Source: three-view drawing plus pictorial views. Frame: mm from the lowest corner of the part. A direction names the side the tool comes from. Give positions to 0.01 mm unless a question says otherwise; leave off trailing zeros. Write each loop counter-clockwise with the first axis right and the second up, starting at its lowest first coordinate (ties: lowest second). Pieces come first, ordered by that corner, then holes. Notation, with made-up numbers: (-12.5, -9.75) - (30.5, -9.75) arc R20 ccw to (30.5, 26.25) - close; hole circle Ø1 at (56, 11.5). An arc over 180 degrees is marked (long way). One line per question, with ' | ' between items. Start each with the question number.
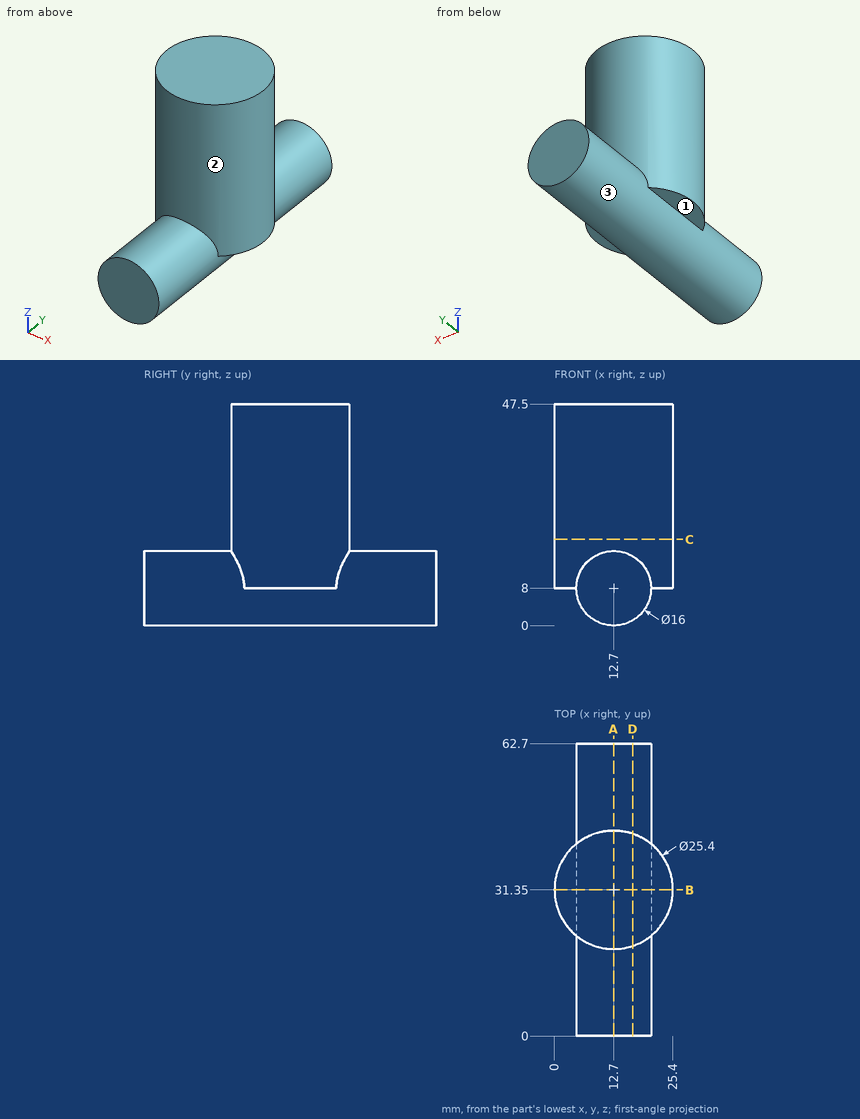
1) First-contact query: pin 1 Ø1.4 at (x, y) = (24, 28.5) entering from -Z; pin 2 Ø1.5 at (x, z) = (3.5, 24) entering from +Y; pin 3 Ø1.5 at (x, z) = (19, 16.5) entering from +Y. Flat tips, straight axial feed; report the tip coordinate or a pass-through.
2) Section B-B, the plane y = 31.35. Output: boundary loops of the cut face in (x, z), plus the area to 3 significant figures.
3) Reachability of the marked faces 1, 2 and 3 from +Z, -Z, +X, -X, +Y, -Y: full face, straight path, thin tool, end or side. Return the list, or none.
4) Section A-A, the plane x = 12.7. Output: boundary loops of the cut face in (y, z).
5) Section C-C, the plane z = 18.5. Output: boundary loops of the cut face in (x, y).
6) Section D-D, the plane x = 16.75. Output: boundary loops of the cut face in (y, z).
7) Line query: L1, parallel to X at y = 31.5, z = 11; L2, parallel to Y at x = 20.25, z = 41; L3, parallel to Z at x = 9, y = 45.5. Output: solid intervals per line, ascending.
Answer key:
1) pin 1: z = 8 | pin 2: y = 40.83 | pin 3: y = 42.77
2) outline: (0, 8) - (4.7, 8) arc R8 ccw to (20.7, 8) - (25.4, 8) - (25.4, 47.5) - (0, 47.5) - close | area: 1,100 mm^2
3) face 1: -Z, -X, +Y, -Y | face 2: +Z | face 3: none
4) outline: (0, 0) - (62.7, 0) - (62.7, 16) - (44.05, 16) - (44.05, 47.5) - (18.65, 47.5) - (18.65, 16) - (0, 16) - close
5) outline: circle Ø25.4 at (12.7, 31.35)
6) outline: (0, 1.1) - (62.7, 1.1) - (62.7, 14.9) - (43.39, 14.9) - (43.39, 47.5) - (19.31, 47.5) - (19.31, 14.9) - (0, 14.9) - close
7) L1: 0 to 25.4 | L2: 21.14 to 41.56 | L3: 0.91 to 15.09
